from build123d import *

# Parameters (mm, degrees)
EXTRUDE_1_DEPTH     = 18
FILLET_1_R          = 2
SKETCH_2_R          = 4.25
CUT_EXTRUDE_1_DEPTH = 49.052055107


with BuildPart() as part:
    # Эскиз1 → Бобышка-Вытянуть1 (new body)
    with BuildSketch(Plane(origin=(0, 0, 0), x_dir=(1, 0, 0), z_dir=(0, 1, 0))):
        with BuildLine():
            Line((0, 14), (0, -14))
            ThreePointArc((0, -14), (0.585786438, -15.414213562), (2, -16))
            Line((2, -16), (31, -16))
            Line((31, -16), (31, -11))
            Line((31, -11), (5, -11))
            Line((5, -11), (5, 11))
            Line((5, 11), (31, 11))
            Line((31, 11), (31, 16))
            Line((31, 16), (2, 16))
            ThreePointArc((2, 16), (0.585786438, 15.414213562), (0, 14))
        make_face()
    extrude(amount=EXTRUDE_1_DEPTH)

    # Скругление1
    fillet_1_edges = [part.edges().sort_by_distance(p)[0] for p in [
        (31, 18, 13.5),
        (31, 0, -13.5),
        (31, 0, 13.5),
        (31, 18, -13.5),
    ]]
    fillet(fillet_1_edges, radius=FILLET_1_R)

    # Эскиз2 → Вырез-Вытянуть1 (cut, through all)
    with BuildSketch(Plane.XY.offset(16)):
        with Locations((22, 9)):
            Circle(SKETCH_2_R)
    extrude(amount=-CUT_EXTRUDE_1_DEPTH, mode=Mode.SUBTRACT)


solid = part.part
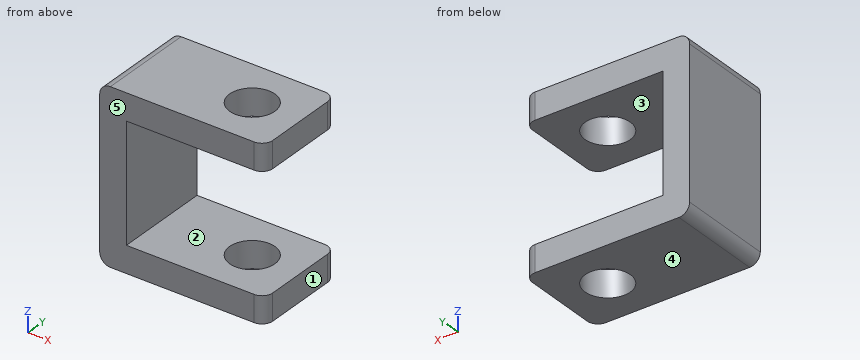
The listing builds one solid part. Answer for the finished solid, in the listing's coordinates (mm). Face numbers are marked on the shaded views. A direction names the side the tool comes from. Give positions to 0.01 mm unless a question says otherwise; leave off trailing zeros. Write each loop counter-clockwise with the first axis right and the second up, starting at its lowest first coordinate (ties: lowest second). Pieces come first, ordered by that corner, then holes. Notation, with made-up numbers: (-11, 6.25) - (19, 6.25) arc R34 ccw to (19, 44.25) - close; hole circle Ø6 at (71, 34). An arc over 180 degrees is marked (long way). One line per question, with ' | ' between items. Start each with the question number.
1. Determine the mould class of the marked faces 3, 4 and 5 for opening direction Z: +Z half, -Z half, draft (parallel to the pull), parting line (faces both ways), or undercut.
2. Given P1, Ø6, axis at x = 22.5, z = -5.5, coming from the -Y side, flat-ended and moving along its own axis, determine where the tip first touches the part or whether it passes through.
3. Section A-A, the plane x = 7 is taken. Determine the outline of the cut face in (y, z), then the cut area to 3 significant figures.
4. For the marked faces 1 and 2, determine the directions among +Z, -Z, +X, -X, +Y, -Y from which every point of the face is accessible in a straight line to the end or side of a thin tool.
5. Straight lines are drawn through the part: line 1 (Z direction, x = 13.5, y = 8.5); line 2 (Y direction, x = 22, z = -12.35); line 3 (X direction, y = 3, z = 8.5). For each, find the intervals that lie inside material, in ascending order.
6. Section D-D, the plane y = 9 is taken. Determine the outline of the cut face in (x, z).
7. Section B-B, the plane z = 11.5 is taken. Determine the outline of the cut face in (x, y), then the cut area to 3 significant figures.
8. Section C-C, the plane x = 22 is taken. Determine the outline of the cut face in (y, z).
Result:
1) face 3: undercut | face 4: -Z half | face 5: draft
2) P1: passes through
3) outline: (0, -16) - (18, -16) - (18, -11) - (0, -11) - close; (0, 11) - (18, 11) - (18, 16) - (0, 16) - close | area: 180 mm2
4) face 1: +Z, -Z, +X, +Y, -Y | face 2: +X, +Y, -Y
5) line 1: z = -16 to -11, 11 to 16 | line 2: y = 0 to 4.75, 13.25 to 18 | line 3: x = 0 to 5
6) outline: (0, -14) arc R2 ccw to (2, -16) - (17.75, -16) - (17.75, -11) - (5, -11) - (5, 11) - (17.75, 11) - (17.75, 16) - (2, 16) arc R2 ccw to (0, 14) - close; (26.25, -16) - (31, -16) - (31, -11) - (26.25, -11) - close; (26.25, 11) - (31, 11) - (31, 16) - (26.25, 16) - close
7) outline: (0, 0) - (29, 0) arc R2 ccw to (31, 2) - (31, 16) arc R2 ccw to (29, 18) - (0, 18) - close; hole circle Ø8.5 at (22, 9) | area: 500 mm2
8) outline: (0, -16) - (4.75, -16) - (4.75, -11) - (0, -11) - close; (0, 11) - (4.75, 11) - (4.75, 16) - (0, 16) - close; (13.25, -16) - (18, -16) - (18, -11) - (13.25, -11) - close; (13.25, 11) - (18, 11) - (18, 16) - (13.25, 16) - close
